Design review of the part built by this model. Coordinates are the model's own, in mm. A direction names the side the tool comes from. Round coordinates to 2 decimals unless told otherwise and drop trailing zeros. Loops run counter-clockwise (first coordinate to the right, second up) from the corner with the lowest first, then second, coordinate; pieces in that order, holes last. Notation, with made-up numbers: M 28,87 L 85,87 A29 ccw 85,125 Z; hole C 79.5,-14.75 d6. An arc over 180 degrees is marked long. One line per item, written item: value. Start each with the question number.
Item 1: For faces 4 (the flat face through (30, 53, -100)), 5 (the flat face through (30, 48, -125)), list the 3-axis set-ups (+Z, -Z, +X, -X, +Y, -Y) from which the entire face can be reached by the end or side of a thin tool; tool diameter is ignored.
Item 2: We need section D-D (z = -103). Write out the cut boundary in (x, y).
Item 3: For line 1 along X through (y, z) = (2, -50); line 2 along Y through (x, z) = (30, -116); line 3 along Z through (x, y) = (14, 15.5), list the stretches that pass through material, from the lowest coordinate up.
Item 4: Mouldability with a two-part tool opening along X and no side actions: class faces 1 (the flat face through (60, 8, -91)), 2 (the cylindrical face through (31.24, 73.42, -112.68)), 3 (the flat face through (23, 10, -51)) as released by +X, released by -X, zero draft, split by the parting line, or undercut.
Item 5: We need section A-A (x = 30). Write out the cut boundary in (y, z).
Item 6: We need section C-C (y = 61). Write out the cut boundary in (x, z), then the cut area to 3 significant figures.
Item 7: Clearance check with flat-ended pins moving along their axes: pin 1 (5 mm diameter, centred on x = 30, z = -50, fed in from +Y); pin 2 (4 mm diameter, centred on y = 35.5, z = -101, fed in from -X); pin 3 (1.5 mm diameter, centred on x = 50, y = 19, fed in from +Z); pin 4 (1 mm diameter, centred on x = 38, z = -32.5, fed in from +Y). State where each tip first meets the part, or that it passes through.
Item 8: We need section B-B (z = -50). Write out the cut boundary in (x, y).
from build123d import *

# Parameters (mm, degrees)
SKETCH1_W           = 60
SKETCH1_H           = 125
BOSS_EXTRUDE1_DEPTH = 10
SKETCH2_R           = 9.5
BOSS_EXTRUDE2_DEPTH = 25
CUT_EXTRUDE1_REACH  = 164.114
SKETCH3_R           = 2.75


with BuildPart() as part:
    # Sketch1 → Boss-Extrude1 (new body)
    with BuildSketch(Plane(origin=(0, 0, 0), x_dir=(1, 0, 0), z_dir=(0, 1, 0))):
        with Locations((30, 62.5)):
            Rectangle(SKETCH1_W, SKETCH1_H)
    extrude(amount=BOSS_EXTRUDE1_DEPTH)

    # Sketch2 → Boss-Extrude2 (add)
    with BuildSketch(Plane(origin=(0, 0, -125), x_dir=(-1, 0, 0), z_dir=(0, 0, -1))):
        with BuildLine():
            Line((-60, 10), (0, 10))
            Line((0, 10), (0, 64))
            ThreePointArc((0, 64), (-30, 94), (-60, 64))
            Line((-60, 64), (-60, 10))
        make_face()
        with Locations((-30, 64)):
            Circle(SKETCH2_R, mode=Mode.SUBTRACT)
    extrude(amount=-BOSS_EXTRUDE2_DEPTH)

    # Sketch3 → Cut-Extrude1 (cut, up to next)
    with BuildSketch(Plane(origin=(0, 10, 0), x_dir=(1, 0, 0), z_dir=(0, 1, 0)), mode=Mode.PRIVATE) as cut_extrude1_sk1:
        with Locations(Location((30, 50, 0), (0, 0, 270))):
            Circle(SKETCH3_R)
    cut_extrude1_tool1 = extrude(cut_extrude1_sk1.sketch, amount=-CUT_EXTRUDE1_REACH, mode=Mode.PRIVATE) & part.part
    add(cut_extrude1_tool1.solids().sort_by_distance((30, 10, -50))[0], mode=Mode.SUBTRACT)


solid = part.part
A:
1. face 4: +Z, +X, -X, +Y
1. face 5: -Z, +X, -X, +Y, -Y
2. outline: M 0,0 L 60,0 L 60,64 A30 ccw 0,64 Z; hole C 30,64 d19
3. line 1: 0 to 27.25, 32.75 to 60
3. line 2: 0 to 54.5, 73.5 to 94
3. line 3: -125 to -100
4. face 1: released by +X
4. face 2: undercut
4. face 3: zero draft
5. outline: M 0,-125 L 54.5,-125 L 54.5,-100 L 10,-100 L 10,-52.75 L 0,-52.75 Z; M 0,-47.25 L 10,-47.25 L 10,0 L 0,0 Z; M 73.5,-125 L 94,-125 L 94,-100 L 73.5,-100 Z
6. outline: M 0,-125 L 20.99,-125 L 20.99,-100 L 0,-100 Z; M 39.01,-125 L 60,-125 L 60,-100 L 39.01,-100 Z
6. area: 1,050 mm2
7. pin 1: through
7. pin 2: x = 0
7. pin 3: z = -100
7. pin 4: y = 10
8. outline: M 0,0 L 27.25,0 L 27.25,10 L 0,10 Z; M 32.75,0 L 60,0 L 60,10 L 32.75,10 Z
